Could you check a few things on this model? Use its own coordinates, in mm. A direction names the side the tool comes from. Round coordinates to 2 decimals unless told otherwise and drop trailing zeros. Write each loop counter-clockwise with the first axis right and the second up, starting at its lowest first coordinate (ties: lowest second). Pieces come first, ordered by that corner, then holes. Notation, with made-up numbers: (35, 2.25) -> (79, 2.25) arc R16 ccw to (79, 33.25) -> close; hole circle Ø6 at (76, 71). An arc over 180 degrees is marked (long way). Answer in a Markdown table with one row per item. Add a question column.
```python
from build123d import *
from OCP.BRepFilletAPI import BRepFilletAPI_MakeChamfer

# Parameters (mm, degrees)
SKETCH1_W           = 5.5
SKETCH1_H           = 2
BOSS_EXTRUDE1_DEPTH = 37
BOSS_EXTRUDE2_START = 35
SKETCH1_3_W         = 5.5
SKETCH1_3_H         = 6.25
BOSS_EXTRUDE2_DEPTH = 2
BOSS_EXTRUDE3_START = 31
SKETCH1_4_W         = 5.5
SKETCH1_4_H         = 6.25
BOSS_EXTRUDE3_DEPTH = 2
BOSS_EXTRUDE5_START = 16
BOSS_EXTRUDE5_DEPTH = 15
SKETCH2_W           = 2
SKETCH2_H           = 5.5
BOSS_EXTRUDE6_DEPTH = 5
SKETCH3_W           = 0.9
SKETCH3_H           = 12.159990002
CUT_EXTRUDE1_DEPTH  = 18.5
CHAMFER1_SIZE2      = 2
CHAMFER1_SIZE       = 1.400415076
CHAMFER2_SIZE       = 2
CHAMFER2_SIZE2      = 1.400415076


with BuildPart() as part:
    # Sketch1 → Boss-Extrude1 (new body)
    with BuildSketch(Plane(origin=(0, 0, 0), x_dir=(0, 0, -1), z_dir=(1, 0, 0))):
        with Locations((2.75, 7.25)):
            Rectangle(SKETCH1_W, SKETCH1_H)
    extrude(amount=BOSS_EXTRUDE1_DEPTH)

    # Sketch1<3> → Boss-Extrude2 (add)
    with BuildSketch(Plane(origin=(0, 0, 0), x_dir=(0, 0, -1), z_dir=(1, 0, 0)).offset(BOSS_EXTRUDE2_START)):
        with Locations((2.75, 3.125)):
            Rectangle(SKETCH1_3_W, SKETCH1_3_H)
    extrude(amount=BOSS_EXTRUDE2_DEPTH)

    # Sketch1<4> → Boss-Extrude3 (add)
    with BuildSketch(Plane(origin=(0, 0, 0), x_dir=(0, 0, -1), z_dir=(1, 0, 0)).offset(BOSS_EXTRUDE3_START)):
        with Locations((2.75, 3.125)):
            Rectangle(SKETCH1_4_W, SKETCH1_4_H)
    extrude(amount=BOSS_EXTRUDE3_DEPTH)

    # Sketch1<6> → Boss-Extrude5 (add)
    with BuildSketch(Plane(origin=(0, 0, 0), x_dir=(0, 0, -1), z_dir=(1, 0, 0)).offset(BOSS_EXTRUDE5_START)):
        with BuildLine():
            Line((0, 1), (0, 0))
            ThreePointArc((0, 0), (2.75, -2.75), (5.5, 0))
            Line((5.5, 0), (5.5, 6.25))
            Line((5.5, 6.25), (4.5, 6.25))
            Line((4.5, 6.25), (4.5, 0))
            ThreePointArc((4.5, 0), (2.75, -1.75), (1, 0))
            Line((1, 0), (1, 1))
            Line((1, 1), (0, 1))
        make_face()
    extrude(amount=BOSS_EXTRUDE5_DEPTH)

    # Sketch2 → Boss-Extrude6 (add)
    with BuildSketch(Plane(origin=(0, 8.25, 0), x_dir=(1, 0, 0), z_dir=(0, 1, 0))):
        with Locations((18.5, 2.75)):
            Rectangle(SKETCH2_W, SKETCH2_H)
    extrude(amount=BOSS_EXTRUDE6_DEPTH)

    # Sketch3 → Cut-Extrude1 (cut)
    with BuildSketch(Plane(origin=(37, 0, 0), x_dir=(0, 0, -1), z_dir=(1, 0, 0))):
        with Locations((3.95, 7.579995001)):
            Rectangle(SKETCH3_W, SKETCH3_H)
    extrude(amount=-CUT_EXTRUDE1_DEPTH, mode=Mode.SUBTRACT)

    # Chamfer1
    chamfer1_edges = [part.edges().sort_by_distance(p)[0] for p in [
        (31, 1.5, -3.95),
    ]]
    chamfer1_side = [part.faces().sort_by_distance(p)[0] for p in [
        (31, 1.471991698, -3.95),
    ]]
    chamfer(chamfer1_edges, length=CHAMFER1_SIZE - 0.0001, length2=CHAMFER1_SIZE2 - 0.0001, reference=chamfer1_side[0])  # a hair under: the kernel refuses the full size

    # Chamfer2: one chamfer whose edges measure the first distance from different faces: ONE call of the kernel's chamfer builder (chamfer() names one face for all edges)
    chamfer2_edges_1 = [part.edges().sort_by_distance(p)[0] for p in [
        (19.5, 8.25, -1.75),
    ]]
    chamfer2_side_1 = [part.faces().sort_by_distance(p)[0] for p in [
        (28.25, 8.25, -1.75),
    ]]
    chamfer2_edges_2 = [part.edges().sort_by_distance(p)[0] for p in [
        (19.5, 8.25, -4.95),
    ]]
    chamfer2_side_2 = [part.faces().sort_by_distance(p)[0] for p in [
        (28.25, 8.25, -4.95),
    ]]
    chamfer2 = BRepFilletAPI_MakeChamfer(part.part.solid().wrapped)
    for e in chamfer2_edges_1:
        chamfer2.Add(CHAMFER2_SIZE, CHAMFER2_SIZE2, e.wrapped, chamfer2_side_1[0].wrapped)  # the first distance lies on this face
    for e in chamfer2_edges_2:
        chamfer2.Add(CHAMFER2_SIZE, CHAMFER2_SIZE2, e.wrapped, chamfer2_side_2[0].wrapped)  # the first distance lies on this face
    add(Compound.cast(chamfer2.Shape()), mode=Mode.REPLACE)


solid = part.part
```
(1) Suppose I cut it at C-C, the plane z = -2.75. Please give me the cut outline in (x, y), then the cut area to 3 significant figures.
(2) On a 3-axis mill with a long thin cutter (end or side, diameter ignored), from which of +Z, -Z, +X, -X, +Y, -Y can I reach the whole of each face in a straight line? I mean faces 4 (the face through (29, 8.25, -2)), 5 (the face through (23.4, -1.75, -2.79)), 6 (the face through (23.4, 0.5, -1)), 7 (the face through (18.5, 10, -4)), 8 (the face through (23.4, 1, -0.5)). Say none if no direction works.
(3) I need wall thicknesses on L1, parallel to X at y = 3.25, z = -3.15; L2, parallel to Y at x = 30, z = -2.75; L3, parallel to X at y = 0.25, z = -0.45. Which ranges of each line are inside material? Lowest first, please.
(4) If we mould it in two halves opening along Z, with no side actions, what happens to faces 1 (the face through (36, 1.5, -4)), 2 (the face through (31, -2, -3)), 3 (the face through (23, 7, 0))? For each: pulls with the +Z half, pulls with the -Z half, needs draft (parallel to the pull), parting line crosses it, or undercut.
(5) For P1, Ø0.5, axis at y = 12, z = -5, coming from the +X side; P2, Ø1.1, axis at x = 21.5, z = -0.5, coming from the +Y side; P3, Ø2, axis at x = 29, z = -2, coming from the +Y side; P4, Ø1, axis at y = 8.5, z = -3.5, coming from the +X side, each with a flat end and sliding along its axis, tell me the tip position at first contact or that it passes through.
(6) Suppose I cut it at A-A, the plane y = 2. Please give me the cut outline in (x, z).
(7) Suppose I cut it at B-B, the plane x = 26. Please give me the cut outline in (y, z).
(8) Suppose I cut it at D-D, the plane y = 7.5. Please give me the cut outline in (x, z).
Response:
| question | item | result |
|---|---|---|
| 1 | outline | (0, 6.25) -> (31, 6.25) -> (31, 0) -> (33, 0) -> (33, 6.25) -> (35, 6.25) -> (35, 0) -> (37, 0) -> (37, 8.25) -> (21.5, 8.25) -> (19.5, 9.65) -> (19.5, 13.25) -> (17.5, 13.25) -> (17.5, 8.25) -> (0, 8.25) -> close; (16, -2.75) -> (31, -2.75) -> (31, -1.75) -> (16, -1.75) -> close |
| 1 | area | 125 mm² |
| 2 | face 4 | +Z, -Z, +X, +Y |
| 2 | face 5 | +X, -X |
| 2 | face 6 | -X |
| 2 | face 7 | +X, +Y |
| 2 | face 8 | +Z, -X |
| 3 | L1 | 31 to 33, 35 to 37 |
| 3 | L2 | -2.75 to -1.75, 6.25 to 8.25 |
| 3 | L3 | 16 to 33, 35 to 37 |
| 4 | face 1 | undercut |
| 4 | face 2 | needs draft |
| 4 | face 3 | pulls with the +Z half |
| 5 | P1 | x = 19.5 |
| 5 | P2 | y = 8.64 |
| 5 | P3 | y = 8.25 |
| 5 | P4 | x = 37 |
| 6 | outline | (16, -5.5) -> (33, -5.5) -> (33, -4.4) -> (31, -4.4) -> (31, -4.5) -> (16, -4.5) -> close; (31, -3.5) -> (33, -3.5) -> (33, 0) -> (31, 0) -> close; (35, -5.5) -> (37, -5.5) -> (37, -4.4) -> (35, -4.4) -> close; (35, -3.5) -> (37, -3.5) -> (37, 0) -> (35, 0) -> close |
| 7 | outline | (0, -5.5) -> (8.25, -5.5) -> (8.25, -4.4) -> (6.25, -4.4) -> (6.25, -4.5) -> (0, -4.5) arc R1.75 cw to (0, -1) -> (1, -1) -> (1, 0) -> (0, 0) arc R2.75 ccw to start; (6.25, -3.5) -> (8.25, -3.5) -> (8.25, 0) -> (6.25, 0) -> close |
| 8 | outline | (0, -5.5) -> (37, -5.5) -> (37, -4.4) -> (18.5, -4.4) -> (18.5, -3.5) -> (37, -3.5) -> (37, 0) -> (0, 0) -> close |
